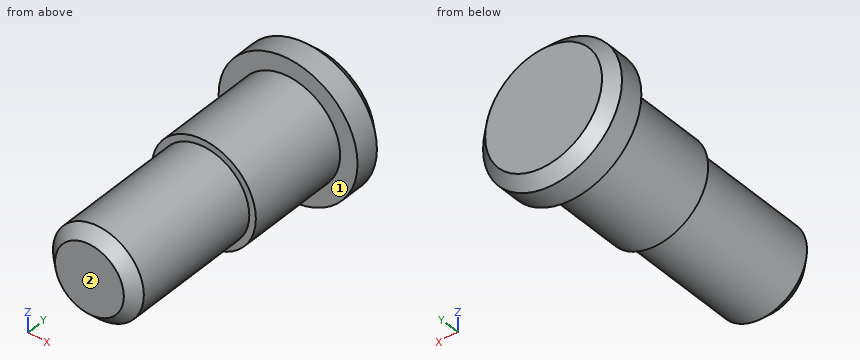
```python
from build123d import *

# Parameters (mm, degrees)
F0_R     = 2.9972
F0_R_2   = 2.61701
F1_DEPTH = 7.9756
F0_R_3   = 4.0005
F2_DEPTH = 2.0066
F3_DEPTH = 16.0782
F4_SIZE  = 0.635


with BuildPart() as f1:
    # F0 (on Front) → F1 (new body)
    with BuildSketch(Plane.XZ):
        Circle(F0_R)
        Circle(F0_R_2, mode=Mode.SUBTRACT)
    extrude(amount=F1_DEPTH)

    # F0 (on Front) → F2 (join)
    with BuildSketch(Plane.XZ):
        Circle(F0_R_3)
        Circle(F0_R, mode=Mode.SUBTRACT)
    extrude(amount=F2_DEPTH)

    # F0 (on Front) → F3 (join)
    with BuildSketch(Plane.XZ):
        Circle(F0_R_2)
    extrude(amount=F3_DEPTH)

    # F4
    f4_edges = [f1.edges().sort_by_distance(p)[0] for p in [
        (-4.0005, 0, 0),
        (-2.61701, -16.0782, 0),
    ]]
    chamfer(f4_edges, length=F4_SIZE)


solid = f1.part
```
Geometry check sheet. Reference: the model listing, model coordinates, mm. Face numbers are marked on the shaded views. A direction names the side the tool comes from. Coordinates: 2 decimals unless noted, no trailing zeros. Order: outer loops, then holes, each group sorted by start corner. A loop starts at its lowest first (then second) coordinate and runs counter-clockwise, first axis right, second up. Notation, with made-up numbers: (17, 67.5) - (43, 67.5) arc R30 ccw to (43, 95.5) - close; hole circle Ø6 at (48.25, 85.25). An arc over 180 degrees is marked (long way). Answer as a JSON object with one key per item and string values. Group by question number.
Item 1: Sectioned sample at D-D, the plane y = -6.5. Record the cut outline in (x, z), and give its area (3 significant figures).
Item 2: Tool access check on the marked faces 1 and 2. Record the directions out of +Z, -Z, +X, -X, +Y, -Y that give a thin tool (end or side, any length) a straight path to the whole face; none if there is none.
Item 3: Scan lines: probe 1 along Y at (x, z) = (0.5, 3.25); probe 2 along Y at (x, z) = (-2.5, 1.5); probe 3 along Z at (x, y) = (-1.5, -2.5). Record each from-to range of solid material in increasing order.
Item 4: Sectioned sample at C-C, the plane y = -10.25. Record the cut outline in (x, z), and give its area (3 significant figures).
Item 5: Depth check by flat-ended pin: pin 1 Ø3 at (x, y) = (0.5, -7.5) entering from +Z; pin 2 Ø1 at (y, z) = (-7.5, -2) entering from +X; pin 3 Ø3 at (x, y) = (2.5, -2) entering from +Z. Enter the tip coordinate at first touch or a pass-through.
Resolved:
{
 "1": {"outline": "circle Ø5.99 at (0, 0)", "area": "28.2 mm^2"},
 "2": {"face 1": "-Y", "face 2": "+Z, -Z, +X, -X, -Y"},
 "3": {"probe 1": "-2.01 to 0", "probe 2": "-7.98 to 0", "probe 3": "-2.59 to 2.59"},
 "4": {"outline": "circle Ø5.23 at (0, 0)", "area": "21.5 mm^2"},
 "5": {"pin 1": "z = 3", "pin 2": "x = 2.59", "pin 3": "z = 3.87"}
}
